For this review, take the finished solid that the model builds, in its own axes (mm). Face numbers are marked on the shaded views. Coordinates: 2 decimals unless noted, no trailing zeros. Order: outer loops, then holes, each group sorted by start corner. A loop starts at its lowest first (then second) coordinate and runs counter-clockwise, first axis right, second up. Notation, with made-up numbers: (3, 59.5) - (39, 59.5) arc R11 cw to (39, 78.5) - close; hole circle Ø1 at (52, 5.25). An arc over 180 degrees is marked (long way). One line per item, written item: value. Start each with the question number.
(1) Consider section C-C on x = -135. Write out the cut boundary in (y, z), then the cut area to 3 significant figures.
(2) Consider section A-A on z = 64. Write out the cut boundary in (x, y).
(3) Clearance check with flat-ended pins moving along their axes: pin 1 (10 mm diameter, centred on x = -166, z = 145, fed in from -Y); pin 2 (3 mm diameter, centred on x = 104.5, y = 43.5, fed in from -Z). State where each tip first meets the part, or that it passes through.
(4) Mouldability with a two-part tool opening along Z and no side actions: class the marked faces 1 and 2 as released by +Z, released by -Z, zero draft, split by the parting line, or undercut.
(5) Consider section B-B on y = 15.5. Write out the cut boundary in (x, z).
(6) To check wall thickness, follow line 1 along Z through (x, y) = (112, 20); line 2 along X through (y, z) = (11, -51.5); line 3 along Y through (x, z) = (228.5, 189). State the ranges of each line that lie inside material, in increasing order.
```python
from build123d import *

# Parameters (mm, degrees)
SKETCH1_W           = 644.525
SKETCH1_H           = 492.125
SKETCH1_W_2         = 635
SKETCH1_H_2         = 482.6
BOSS_EXTRUDE1_DEPTH = 50.8
SKETCH2_W           = 492.125
SKETCH2_H           = 4.7625
BOSS_EXTRUDE2_DEPTH = 644.525
FILLET1_R           = 10.16


with BuildPart() as part:
    # Sketch1 → Boss-Extrude1 (new body)
    with BuildSketch(Plane(origin=(0, 0, 0), x_dir=(1, 0, 0), z_dir=(0, 1, 0))):
        Rectangle(SKETCH1_W, SKETCH1_H)
        Rectangle(SKETCH1_W_2, SKETCH1_H_2, mode=Mode.SUBTRACT)
    extrude(amount=BOSS_EXTRUDE1_DEPTH)

    # Sketch2 → Boss-Extrude2 (add)
    with BuildSketch(Plane(origin=(322.2625, 0, 0), x_dir=(0, 0, -1), z_dir=(1, 0, 0))):
        with Locations((0, 48.41875)):
            Rectangle(SKETCH2_W, SKETCH2_H)
    extrude(amount=-BOSS_EXTRUDE2_DEPTH)

    # Fillet1
    fillet1_edges = [part.edges().sort_by_distance(p)[0] for p in [
        (-322.2625, 50.8, 0),
        (0, 50.8, 246.0625),
        (322.2625, 50.8, 0),
        (0, 50.8, -246.0625),
        (322.2625, 25.4, 246.0625),
        (-322.2625, 25.4, 246.0625),
        (-322.2625, 25.4, -246.0625),
        (322.2625, 25.4, -246.0625),
    ]]
    fillet(fillet1_edges, radius=FILLET1_R)


solid = part.part
```
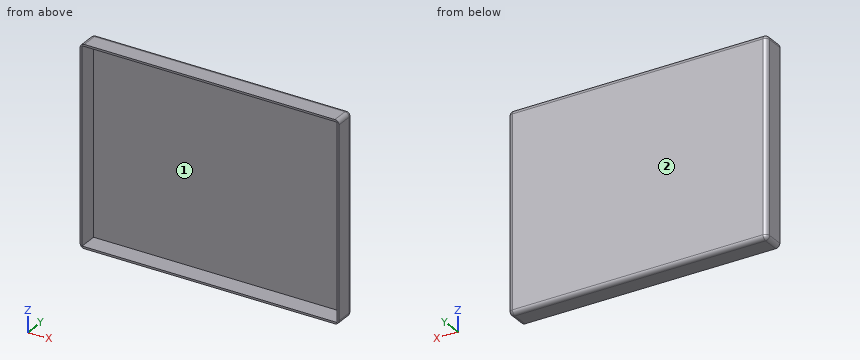
Geometry check:
1. outline: (0, -246.06) - (40.64, -246.06) arc R10.16 ccw to (50.8, -235.9) - (50.8, 235.9) arc R10.16 ccw to (40.64, 246.06) - (0, 246.06) - (0, 241.3) - (46.04, 241.3) - (46.04, -241.3) - (0, -241.3) - close
1. area: 2,740 mm^2
2. outline: (-322.26, 0) - (-317.5, 0) - (-317.5, 46.04) - (317.5, 46.04) - (317.5, 0) - (322.26, 0) - (322.26, 40.64) arc R10.16 ccw to (312.1, 50.8) - (-312.1, 50.8) arc R10.16 ccw to (-322.26, 40.64) - close
3. pin 1: stops at y = 46.04
3. pin 2: stops at z = -245.97
4. face 1: undercut
4. face 2: zero draft
5. outline: (-322.26, -235.9) arc R10.16 ccw to (-312.1, -246.06) - (312.1, -246.06) arc R10.16 ccw to (322.26, -235.9) - (322.26, 235.9) arc R10.16 ccw to (312.1, 246.06) - (-312.1, 246.06) arc R10.16 ccw to (-322.26, 235.9) - close; hole (-317.5, -241.3) - (317.5, -241.3) - (317.5, 241.3) - (-317.5, 241.3) - close
6. line 1: z = -246.06 to -241.3, 241.3 to 246.06
6. line 2: x = -322.26 to -317.5, 317.5 to 322.26
6. line 3: y = 46.04 to 50.8
